Source: CAD feature listing. Evaluate the final solid. Frame: model axes, mm. A direction names the side the tool comes from. Give positions to 0.01 mm unless a question says otherwise; leave off trailing zeros. Order: outer loops, then holes, each group sorted by start corner. A loop starts at its lowest first (then second) coordinate and runs counter-clockwise, first axis right, second up. Notation, with made-up numbers: (-7.75, 60) -> (13.25, 60) arc R17 cw to (13.25, 65) -> close; hole circle Ø10 at (22, -6). An arc over 180 degrees is marked (long way). Answer in a Markdown table with one row per item.
```python
from build123d import *

# Parameters (mm, degrees)
BOSS_EXTRUDE1_DEPTH = 38.1
BOSS_EXTRUDE2_DEPTH = 25.4
CUT_EXTRUDE1_DEPTH  = 2.921
SKETCH5_R           = 3.2385
CUT_EXTRUDE3_DEPTH  = 58.589283942


with BuildPart() as part:
    # Sketch1 → Boss-Extrude1 (new, symmetric)
    with BuildSketch(Plane(origin=(0, 0, 0), x_dir=(1, 0, 0), z_dir=(0, 1, 0))):
        with BuildLine():
            Line((-13.928921766, 0), (13.928921766, 0))
            Line((13.928921766, 0), (13.928921766, 12.394153757))
            Line((13.928921766, 12.394153757), (10.753921766, 12.394153757))
            ThreePointArc((10.753921766, 12.394153757), (0, 2.54), (-10.753921766, 12.394153757))
            Line((-10.753921766, 12.394153757), (-13.928921766, 12.394153757))
            Line((-13.928921766, 12.394153757), (-13.928921766, 0))
        make_face()
    extrude(amount=BOSS_EXTRUDE1_DEPTH, both=True)

    # Sketch2 → Boss-Extrude2 (add, symmetric)
    with BuildSketch(Plane(origin=(0, 0, 0), x_dir=(0, 0, -1), z_dir=(1, 0, 0))):
        with BuildLine():
            Line((-18.306045368, -16.053970918), (-18.306045368, -38.1))
            Line((-18.306045368, -38.1), (-25.926045368, -38.1))
            Line((-25.926045368, -38.1), (-25.926045368, -16.005144511))
            ThreePointArc((-25.926045368, -16.005144511), (-34.925, 0), (-25.926045368, 16.005144511))
            Line((-25.926045368, 16.005144511), (-25.926045368, 38.1))
            Line((-25.926045368, 38.1), (2.54, 38.1))
            Line((2.54, 38.1), (2.54, -38.1))
            Line((2.54, -38.1), (-14.078954632, -38.1))
            Line((-14.078954632, -38.1), (-14.078954632, -16.053970918))
            ThreePointArc((-14.078954632, -16.053970918), (-16.1925, 16.1925), (-18.306045368, -16.053970918))
        make_face()
    extrude(amount=BOSS_EXTRUDE2_DEPTH, both=True)

    # Sketch3 → Cut-Extrude1 (cut, symmetric)
    with BuildSketch(Plane.XY.offset(22.116045368)):
        Polygon((5.5245, -28.589571562), (5.5245, -22.210428438), (0, -19.020856876), (-5.5245, -22.210428438), (-5.5245, -28.589571562), (-5.5245, -38.1), (5.5245, -38.1), align=None)
    cut_extrude1 = extrude(amount=CUT_EXTRUDE1_DEPTH, both=True, mode=Mode.SUBTRACT)

    # Sketch5 → Cut-Extrude3 (cut, symmetric)
    with BuildSketch(Plane.XY):
        with Locations(Location((0, -25.4, 0), (0, 0, 180))):
            Circle(SKETCH5_R)
    cut_extrude3 = extrude(amount=CUT_EXTRUDE3_DEPTH, both=True, mode=Mode.SUBTRACT)

    # Mirror1: Cut-Extrude1, Cut-Extrude3 across plane
    add(cut_extrude1.mirror(Plane.ZX), mode=Mode.SUBTRACT)
    add(cut_extrude3.mirror(Plane.ZX), mode=Mode.SUBTRACT)


solid = part.part
```
(1) Section query D-D (x = -18). Return the cut outline in (y, z) (1 decimal).
A:
| item | result |
|---|---|
| outline | (-38.1, -2.5) -> (38.1, -2.5) -> (38.1, 25.9) -> (16, 25.9) arc R18.7 ccw to (-16, 25.9) -> (-38.1, 25.9) -> (-38.1, 18.3) -> (-16.1, 18.3) arc R16.2 cw (long way) to (-16.1, 14.1) -> (-38.1, 14.1) -> close |
(2) Access query for faces 1 (the flat face through (2.801, -20.638, 22.157)), 2 (the flat face through (0, 31, 25.037)), 3 (the flat face through (0, -29, 18.306)). Directions: +Z, -Z, +X, -X, +Y, -Y. A direction counts if a zero-diameter tool reaches every point of the face in a straight line with its end or side. Return the directions, or none.
A:
| item | result |
|---|---|
| face 1 | -Y |
| face 2 | +Y |
| face 3 | +X, -X, -Y |
(3) Section query A-A (y = -25.4). Give the number of separate pieces and of enclosed holes in the cut face, plus the area to 3 significant figures.
A:
| item | result |
|---|---|
| separate pieces | 4 |
| enclosed holes | 0 |
| area | 1,160 mm^2 |
(4) Ray query, probe 1 along Z at (x, y) = (13.5, -25.5); probe 2 along Z at (x, y) = (0, 0) (3 decimals); probe 3 along Y at (x, z) = (0, 25.5). Return the intervals inside material, ascending.
A:
| item | result |
|---|---|
| probe 1 | z = -12.39 to 14.08, 18.31 to 25.93 |
| probe 2 | z = -2.54 to 0, 32.385 to 34.925 |
| probe 3 | y = -38.1 to -28.64, -22.16 to -13.25, 13.25 to 22.16, 28.64 to 38.1 |
(5) First-contact query: pin 1 Ø7.5 at (x, y) = (0, -25.4) entering from +Z; pin 2 Ø10 at (x, y) = (-15.5, -14) entering from -Z; pin 3 Ø9 at (x, y) = (22, 17.5) entering from -Z; pin 4 Ø9 at (x, y) = (3, -29) entering from -Z. Flat tips, straight axial feed; report the tip coordinate or a pass-through.
A:
| item | result |
|---|---|
| pin 1 | stops at z = 25.93 |
| pin 2 | stops at z = -12.39 |
| pin 3 | stops at z = -2.54 |
| pin 4 | stops at z = -5.57 |
(6) Pull-direction query (Y, two-part tool) for faces 4 (the cylindrical face through (0.7, 22.24, 25.49)), 5 (the flat face through (25.4, 1, -1)), 6 (the flat face through (0, 38.1, 11)); classes: +Y half, -Y half, draft (parallel to the pull), parting line (faces both ways), or undercut.
A:
| item | result |
|---|---|
| face 4 | undercut |
| face 5 | draft |
| face 6 | +Y half |
(7) Section query B-B (z = 12.5). Return the cut outline in (x, y).
A:
| item | result |
|---|---|
| outline | (-25.4, -38.1) -> (25.4, -38.1) -> (25.4, -15.77) -> (-25.4, -15.77) -> close; (-25.4, 15.77) -> (25.4, 15.77) -> (25.4, 38.1) -> (-25.4, 38.1) -> close; hole circle Ø6.48 at (0, -25.4); hole circle Ø6.48 at (0, 25.4) |
(8) Section query C-C (y = 0). Return the cut outline in (x, z) (3 decimals), plus the area to 3 significant figures.
A:
| item | result |
|---|---|
| outline | (-25.4, -2.54) -> (-13.929, -2.54) -> (-13.929, -12.394) -> (-10.754, -12.394) arc R10.795 cw to (10.754, -12.394) -> (13.929, -12.394) -> (13.929, -2.54) -> (25.4, -2.54) -> (25.4, 0) -> (-25.4, 0) -> close; (-25.4, 32.385) -> (25.4, 32.385) -> (25.4, 34.925) -> (-25.4, 34.925) -> close |
| area | 370 mm^2 |
